The listing builds one solid part. Answer for the finished solid, in the listing's coordinates (mm). Give positions to 0.01 mm unless a question says otherwise; leave off trailing zeros. Order: outer loops, then holes, each group sorted by start corner. A loop starts at its lowest first (then second) coordinate and runs counter-clockwise, first axis right, second up.
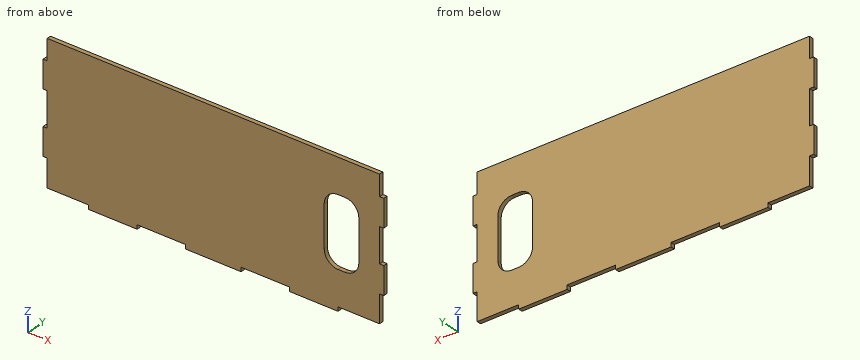
```python
from build123d import *

# Parameters (mm, degrees)
SKETCH2_W           = 240
SKETCH2_H           = 3
BOSS_EXTRUDE1_DEPTH = 100
SKETCH3_W           = 20
SKETCH3_H           = 3
BOSS_EXTRUDE2_DEPTH = 3
BOSS_EXTRUDE3_START = -240
SKETCH3_2_W         = 20
SKETCH3_2_H         = 3
BOSS_EXTRUDE3_DEPTH = 3
SKETCH4_W           = 35
SKETCH4_H           = 3
SKETCH4_W_2         = 40
BOSS_EXTRUDE4_DEPTH = 3
CUT_EXTRUDE1_DEPTH  = 3


with BuildPart() as part:
    # Sketch2 → Boss-Extrude1 (new body)
    with BuildSketch(Plane.XY):
        Rectangle(SKETCH2_W, SKETCH2_H)
    extrude(amount=BOSS_EXTRUDE1_DEPTH)

    # Sketch3 → Boss-Extrude2 (add)
    with BuildSketch(Plane.ZY.offset(120)):
        with Locations((30, 0)):
            Rectangle(SKETCH3_W, SKETCH3_H)
        with Locations((75, 0)):
            Rectangle(SKETCH3_W, SKETCH3_H)
    extrude(amount=BOSS_EXTRUDE2_DEPTH)

    # Sketch3<2> → Boss-Extrude3 (add)
    with BuildSketch(Plane.ZY.offset(120).offset(BOSS_EXTRUDE3_START)):
        with Locations((30, 0)):
            Rectangle(SKETCH3_2_W, SKETCH3_2_H)
        with Locations((75, 0)):
            Rectangle(SKETCH3_2_W, SKETCH3_2_H)
    extrude(amount=-BOSS_EXTRUDE3_DEPTH)

    # Sketch4 → Boss-Extrude4 (add)
    with BuildSketch(Plane(origin=(0, 0, 0), x_dir=(-1, 0, 0), z_dir=(0, 0, -1))):
        with Locations((-72.5, 0)):
            Rectangle(SKETCH4_W, SKETCH4_H)
        Rectangle(SKETCH4_W_2, SKETCH4_H)
        with Locations((72.5, 0)):
            Rectangle(SKETCH4_W, SKETCH4_H)
    extrude(amount=BOSS_EXTRUDE4_DEPTH)

    # Sketch5 → Cut-Extrude1 (cut)
    with BuildSketch(Plane(origin=(0, 1.5, 0), x_dir=(1, 0, 0), z_dir=(0, 1, 0))):
        with BuildLine():
            Line((90, -25), (95, -25))
            ThreePointArc((95, -25), (102.071067812, -27.928932188), (105, -35))
            Line((105, -35), (105, -65))
            ThreePointArc((105, -65), (102.071067812, -72.071067812), (95, -75))
            Line((95, -75), (90, -75))
            ThreePointArc((90, -75), (82.928932188, -72.071067812), (80, -65))
            Line((80, -65), (80, -35))
            ThreePointArc((80, -35), (82.928932188, -27.928932188), (90, -25))
        make_face()
    extrude(amount=-CUT_EXTRUDE1_DEPTH, mode=Mode.SUBTRACT)


solid = part.part
```
1) Find section A-A (z = 45.5). Write down the section's boundary in (x, y), then the cut area to 3 significant figures.
Geometry says:
outline: (-120, -1.5) - (80, -1.5) - (80, 1.5) - (-120, 1.5) - close; (105, -1.5) - (120, -1.5) - (120, 1.5) - (105, 1.5) - close
area: 645 mm2
2) Find section B-B (x = 98). Write down the section's boundary in (y, z).
Geometry says:
outline: (-1.5, 0) - (1.5, 0) - (1.5, 25.46) - (-1.5, 25.46) - close; (-1.5, 74.54) - (1.5, 74.54) - (1.5, 100) - (-1.5, 100) - close
3) Given P1, Ø1.5, axis at x = 121.5, y = 0, coming from the -Z side; P2, Ø1.5, axis at x = 92, y = 0.5, coming from the -Z side; P3, Ø0.9, axis at x = 122, y = 0.5, coming from the +Z side, each flat-ended and moving along its own axis, determine where each tip first touches the part or whether it passes through.
Geometry says:
P1: stops at z = 20
P2: stops at z = 0
P3: stops at z = 85
4) Find section D-D (x = -38.5). Write down the section's boundary in (y, z).
Geometry says:
outline: (-1.5, 0) - (1.5, 0) - (1.5, 100) - (-1.5, 100) - close
5) Straight lines are drawn through the part: probe 1 along X at (y, z) = (-1.05, 64.5); probe 2 along Z at (x, y) = (94, -0.45); probe 3 along X at (y, z) = (0.5, 65.5). For each, find the intervals that lie inside material, in ascending order.
Geometry says:
probe 1: x = -120 to 80, 105 to 120
probe 2: z = 0 to 25, 75 to 100
probe 3: x = -123 to 80.01, 104.99 to 123
6) Find section C-C (z = 7). Write down the section's boundary in (x, y).
Geometry says:
outline: (-120, -1.5) - (120, -1.5) - (120, 1.5) - (-120, 1.5) - close
